from build123d import *

# Parameters (mm, degrees)
BOSS_EXTRUDE1_DEPTH      = 48
SKETCH2_W                = 14
SKETCH2_H                = 10
BOSS_EXTRUDE2_DEPTH      = 50
FILLET1_R                = 6
SKETCH7_R                = 38.5
SKETCH7_R_2              = 35
BOSS_EXTRUDE3_DEPTH      = 10
SKETCH8_R                = 35
CUT_EXTRUDE2_DEPTH       = 90
BOSS_EXTRUDE4_DEPTH      = 5
BOSS_EXTRUDE4_DEPTH_BACK = 10
SKETCH10_R               = 12
SKETCH10_R_2             = 9
BOSS_EXTRUDE5_START      = 25
SKETCH11_R               = 10
SKETCH11_R_2             = 9
BOSS_EXTRUDE5_DEPTH      = 25
SKETCH12_R               = 9
CUT_EXTRUDE3_DEPTH       = 42
BOSS_EXTRUDE6_DEPTH      = 7.5
BOSS_EXTRUDE7_START      = 7.5
BOSS_EXTRUDE7_DEPTH      = 7.5
FILLET1_OF_MIRROR1_R     = 6
SKETCH15_W               = 14
SKETCH15_H               = 10
CUT_EXTRUDE4_DEPTH       = 101
BOSS_EXTRUDE8_DEPTH      = 10


with BuildPart() as part:
    # Sketch1 → Boss-Extrude1 (new body)
    with BuildSketch(Plane.XY):
        with BuildLine():
            Line((0, 0), (0, 25.00039893))
            Line((0, 25.00039893), (22, 25.00039893))
            ThreePointArc((22, 25.00039893), (51.667114877, 29.062120939), (80, 38.751440389))
            Line((80, 38.751440389), (80, 6.798665084))
            ThreePointArc((80, 6.798665084), (51.198552391, 1.705464917), (22, 0))
            Line((22, 0), (0, 0))
        make_face()
    extrude(amount=BOSS_EXTRUDE1_DEPTH)

    # Sketch2 → Boss-Extrude2 (add)
    with BuildSketch(Plane.XY.offset(48)):
        with Locations((11.5, 12.5)):
            Rectangle(SKETCH2_W, SKETCH2_H)
    boss_extrude2 = extrude(amount=BOSS_EXTRUDE2_DEPTH)

    # Sketch5 → M8x1.0 Tapped Hole1 (revolve, cut)
    with BuildSketch(Plane(origin=(11.5, 17.5, 86), x_dir=(0, 0, 1), z_dir=(1, 0, 0))):
        Polygon((0, 0), (0, 12.103012167), (3.5, 10), (3.5, 0), align=None)
    m8x1_0_tapped_hole1 = revolve(axis=Axis((11.5, 23.85, 86), (0, -1, 0)), mode=Mode.SUBTRACT)

    # Fillet1
    fillet1_edges = [part.edges().sort_by_distance(p)[0] for p in [
        (18.5, 12.5, 98),
        (4.5, 12.5, 98),
    ]]
    fillet(fillet1_edges, radius=FILLET1_R)

    # Sketch7 → Boss-Extrude3 (add)
    with BuildSketch(Plane.ZY.offset(-80)):
        with Locations((24, 60.00039893)):
            Circle(SKETCH7_R)
        with Locations((24, 60.00039893)):
            Circle(SKETCH7_R_2, mode=Mode.SUBTRACT)
    extrude(amount=BOSS_EXTRUDE3_DEPTH)

    # Sketch8 → Cut-Extrude2 (cut)
    with BuildSketch(Plane.ZY.offset(-80)):
        with Locations(Location((24, 60.00039893, 0), (0, 0, 226.708192407))):
            Circle(SKETCH8_R)
    extrude(amount=CUT_EXTRUDE2_DEPTH, mode=Mode.SUBTRACT)

    # Sketch10 → Boss-Extrude4 (add, two sides: drawn at the far end of the back side and taken through both)
    with BuildSketch(Plane.XZ.offset(-BOSS_EXTRUDE4_DEPTH_BACK)):
        with Locations((14.5, 24)):
            Circle(SKETCH10_R)
        with Locations((14.5, 24)):
            Circle(SKETCH10_R_2, mode=Mode.SUBTRACT)
    extrude(amount=BOSS_EXTRUDE4_DEPTH + BOSS_EXTRUDE4_DEPTH_BACK)

    # Sketch11 → Boss-Extrude5 (add)
    with BuildSketch(Plane.XZ.offset(5).offset(BOSS_EXTRUDE5_START)):
        with Locations((14.5, 24)):
            Circle(SKETCH11_R)
        with Locations((14.5, 24)):
            Circle(SKETCH11_R_2, mode=Mode.SUBTRACT)
    extrude(amount=-BOSS_EXTRUDE5_DEPTH)

    # Sketch12 → Cut-Extrude3 (cut)
    with BuildSketch(Plane(origin=(0, 0, 0), x_dir=(-1, 0, 0), z_dir=(0, -1, 0))):
        with Locations(Location((-14.5, -24, 0), (0, 0, 180))):
            Circle(SKETCH12_R)
    extrude(amount=-CUT_EXTRUDE3_DEPTH, mode=Mode.SUBTRACT)

    # Sketch13 → Boss-Extrude6 (add)
    with BuildSketch(Plane.XY.offset(48)):
        with BuildLine():
            Line((0, 25.00039893), (0, 0))
            Line((0, 0), (22, 0))
            ThreePointArc((22, 0), (51.198552391, 1.705464917), (80, 6.798665084))
            Line((80, 6.798665084), (80, 29.896412483))
            Line((80, 29.896412483), (80, 34.524920524))
            Line((80, 34.524920524), (70, 34.524920524))
            Line((70, 34.524920524), (69.729925021, 34.524920524))
            ThreePointArc((69.729925021, 34.524920524), (46.24106465, 27.877911315), (22, 25.00039893))
            Line((22, 25.00039893), (0, 25.00039893))
        make_face()
    extrude(amount=BOSS_EXTRUDE6_DEPTH)

    # Sketch14 → Boss-Extrude7 (add)
    with BuildSketch(Plane(origin=(0, 0, 0), x_dir=(-1, 0, 0), z_dir=(0, 0, -1)).offset(BOSS_EXTRUDE7_START)):
        with BuildLine():
            Line((-80, 29.896412483), (-80, 6.798665084))
            ThreePointArc((-80, 6.798665084), (-51.198552391, 1.705464917), (-22, 0))
            Line((-22, 0), (0, 0))
            Line((0, 0), (0, 25.00039893))
            Line((0, 25.00039893), (-22, 25.00039893))
            ThreePointArc((-22, 25.00039893), (-46.24106465, 27.877911315), (-69.729925021, 34.524920524))
            Line((-69.729925021, 34.524920524), (-70, 34.524920524))
            Line((-70, 34.524920524), (-80, 34.524920524))
            Line((-80, 34.524920524), (-80, 29.896412483))
        make_face()
    extrude(amount=-BOSS_EXTRUDE7_DEPTH)

    # Mirror1: Boss-Extrude2, M8x1.0 Tapped Hole1 across plane
    add(boss_extrude2.mirror(Plane.XY.offset(24)))
    add(m8x1_0_tapped_hole1.mirror(Plane.XY.offset(24)), mode=Mode.SUBTRACT)

    # Fillet1 of Mirror1
    fillet1_of_mirror1_edges = [part.edges().sort_by_distance(p)[0] for p in [
        (18.5, 12.5, -50),
        (4.5, 12.5, -50),
    ]]
    fillet(fillet1_of_mirror1_edges, radius=FILLET1_OF_MIRROR1_R)

    # Sketch15 → Cut-Extrude4 (cut)
    with BuildSketch(Plane.XY.offset(61.5)):
        with Locations((11.5, 12.5)):
            Rectangle(SKETCH15_W, SKETCH15_H)
    extrude(amount=CUT_EXTRUDE4_DEPTH, mode=Mode.SUBTRACT)

    # Sketch16 → Boss-Extrude8 (add)
    with BuildSketch(Plane(origin=(80, 0, 0), x_dir=(0, 0, -1), z_dir=(1, 0, 0))):
        with BuildLine():
            Line((-55.5, 75.256545232), (-55.5, 506.798665084))
            Line((-55.5, 506.798665084), (7.5, 506.798665084))
            Line((7.5, 506.798665084), (7.5, 75.256545232))
            ThreePointArc((7.5, 75.256545232), (-24, 95.00039893), (-55.5, 75.256545232))
        make_face()
    extrude(amount=-BOSS_EXTRUDE8_DEPTH)


solid = part.part
Can you work these out from the model? Positions are in its coordinate system, mm. A direction names the side the tool comes from. Coordinates: 2 decimals unless noted, no trailing zeros. Loops run counter-clockwise (first coordinate to the right, second up) from the corner with the lowest first, then second, coordinate; pieces in that order, holes last. Notation, with made-up numbers: (33, 23.25) - (82, 23.25) arc R26 cw to (82, 61.25) - close; hole circle Ø5 at (47, 3.25). An arc over 180 degrees is marked (long way). Put each result on its own line as item: value. Start each with the question number.
Item 1: Which directions (+Z, -Z, +X, -X, +Y, -Y) give clear straight access to the entire face, cutting with the end or side of a thin tool? Please do faces 1 (the face through (11, 7.5, -28)), 2 (the face through (75, 291, 55.5)), 3 (the face through (4, 25, 24)), 4 (the face through (75, 297, -7.5)).
Item 2: For pin 1 (4.5 mm diameter, centred on y = 52.5, z = 57, fed in from -X); pin 2 (8 mm diameter, centred on x = 73, y = 245.5, fed in from -Z); pin 3 (5 mm diameter, centred on x = 8.5, z = 59.5, fed in from +Y), each with a flat end and sliding along its axis, tell me the tip position at first contact or that it passes through.
Item 3: Suppose I cut it at A-A (y = 65). Please give me the cut outline in (x, z).
Item 4: Suppose I cut it at C-C (z = -28.5). Please give me the cut outline in (x, y).
Item 5: If we mould it in two halves opening along Z, with no side actions, what happens to faces 5 (the face through (13.198, -17.675, 33.915)), 6 (the face through (80, 316, 23)), 7 (the face through (23.084, -2.857, 26.703))? For each: +Z half, -Z half, draft (parallel to the pull), parting line (faces both ways), or undercut.
Item 6: If I drill on line 1 along X through (y, z) = (10, -38); line 2 along Z through (x, y) = (14, -12); line 3 along Z through (x, y) = (11.5, 10), over which ranges is the centre line in solid material (lowest first)?
Item 7: Suppose I cut it at D-D (y = 378.5). Please give me the cut outline in (x, z).
Item 8: Suppose I cut it at B-B (x = 44). Please give me the cut outline in (y, z).
Here are the results:
1. face 1: -Z, +X, -X, -Y
1. face 2: +Z, +X, -X, +Y
1. face 3: +Z, -Z, -X, +Y
1. face 4: -Z, +X, -X, +Y
2. pin 1: x = 70
2. pin 2: z = -7.5
2. pin 3: y = 17.5
3. outline: (70, -14.17) - (80, -14.17) - (80, -10.64) - (70, -10.64) - close; (70, 58.64) - (80, 58.64) - (80, 62.17) - (70, 62.17) - close
4. outline: (4.5, 7.5) - (18.5, 7.5) - (18.5, 17.5) - (4.5, 17.5) - close
5. face 5: parting line
5. face 6: draft
5. face 7: undercut
6. line 1: 4.5 to 8, 15 to 18.5
6. line 2: 14.01 to 15.01, 32.99 to 33.99
6. line 3: -50 to -41.5, -34.5 to 15.51, 32.49 to 61.5
7. outline: (70, -7.5) - (80, -7.5) - (80, 55.5) - (70, 55.5) - close
8. outline: (0.97, -7.5) - (27.45, -7.5) - (27.45, 11.14) arc R35 cw to (27.45, 36.86) - (27.45, 55.5) - (0.97, 55.5) - close
